Build history of the part. All positions in model axes, mm. Give positions to 0.01 mm unless a question says otherwise; leave off trailing zeros. Order: outer loops, then holes, each group sorted by start corner. A loop starts at its lowest first (then second) coordinate and runs counter-clockwise, first axis right, second up. Notation, with made-up numbers: (-19, -6.5) - (-2, -6.5) arc R29 cw to (-2, 21.5) - close; hole circle Ø4 at (12, -21). An arc over 180 degrees is marked (long way). Use a Markdown table: item, result.
from build123d import *

# Parameters (mm, degrees)
F0_R     = 34
F1_DEPTH = 0.5


with BuildPart() as f1:
    # F0 (on Top) → F1 (new body)
    with BuildSketch(Plane.XY):
        Circle(F0_R)
        with BuildLine():
            ThreePointArc((-27.595006, 7.125), (-22.1129, 10.357106), (-18.880794, 4.875))
            ThreePointArc((-18.880794, 4.875), (-19.5, 0), (-18.880794, -4.875))
            ThreePointArc((-18.880794, -4.875), (-22.1129, -10.357106), (-27.595006, -7.125))
            ThreePointArc((-27.595006, -7.125), (-28.5, 0), (-27.595006, 7.125))
        make_face(mode=Mode.SUBTRACT)
        with BuildLine():
            ThreePointArc((18.880794, -4.875), (19.5, 0), (18.880794, 4.875))
            ThreePointArc((18.880794, 4.875), (22.1129, 10.357106), (27.595006, 7.125))
            ThreePointArc((27.595006, 7.125), (28.5, 0), (27.595006, -7.125))
            ThreePointArc((27.595006, -7.125), (22.1129, -10.357106), (18.880794, -4.875))
        make_face(mode=Mode.SUBTRACT)
    extrude(amount=F1_DEPTH)


solid = f1.part
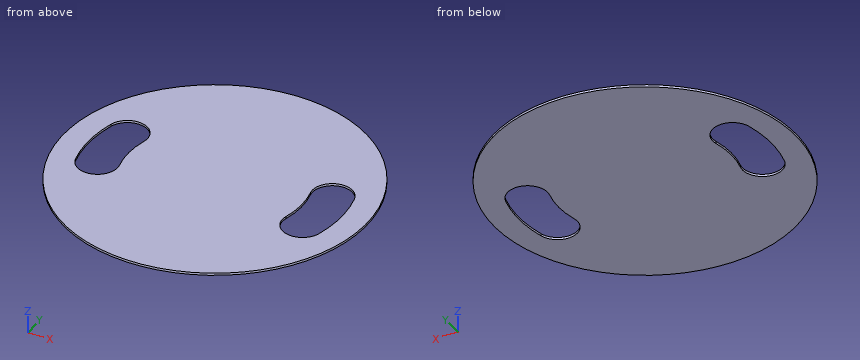
1) Slice it at D-D (x = 24). Write the cut outline in (y, z) (3 decimals), and give its area (3 significant figures).
Computed:
| item | result |
|---|---|
| outline | (-24.083, 0) - (-10.435, 0) - (-10.435, 0.5) - (-24.083, 0.5) - close; (10.435, 0) - (24.083, 0) - (24.083, 0.5) - (10.435, 0.5) - close |
| area | 13.6 mm² |
2) Pin check, flat tip, straight feed: P1, Ø6, axis at x = 19, y = 22.5, coming from the -Z side. Stop position of the tip, or through.
Computed:
| item | result |
|---|---|
| P1 | stops at z = 0 |
3) Slice it at A-A (z = 0.1). Write the cut outline in (x, y) (3 decimals), and give its area (3 significant figures).
Computed:
| item | result |
|---|---|
| outline | circle Ø68 at (0, 0); hole (-27.595, -7.125) arc R4.5 ccw to (-18.881, -4.875) arc R19.5 cw to (-18.881, 4.875) arc R4.5 ccw to (-27.595, 7.125) arc R28.5 ccw to start; hole (18.881, -4.875) arc R4.5 ccw to (27.595, -7.125) arc R28.5 ccw to (27.595, 7.125) arc R4.5 ccw to (18.881, 4.875) arc R19.5 cw to start |
| area | 3,290 mm² |
4) Slice it at C-C (x = -26). Write the cut outline in (y, z), and give its area (3 significant figures).
Computed:
| item | result |
|---|---|
| outline | (-21.91, 0) - (-9.55, 0) - (-9.55, 0.5) - (-21.91, 0.5) - close; (9.55, 0) - (21.91, 0) - (21.91, 0.5) - (9.55, 0.5) - close |
| area | 12.4 mm² |
5) Slice it at B-B (y = 0). Write the cut outline in (x, z).
Computed:
| item | result |
|---|---|
| outline | (-34, 0) - (-28.5, 0) - (-28.5, 0.5) - (-34, 0.5) - close; (-19.5, 0) - (19.5, 0) - (19.5, 0.5) - (-19.5, 0.5) - close; (28.5, 0) - (34, 0) - (34, 0.5) - (28.5, 0.5) - close |
6) Wall check: line 1 (X direction, y = 2, z = 0.4); line 2 (X direction, y = -1, z = 0.1); line 3 (Y direction, x = -25, z = 0.35). Give the ranges that are in metal, low to high. Write a range as from..to.
Computed:
| item | result |
|---|---|
| line 1 | x = -33.94..-28.43, -19.4..19.4, 28.43..33.94 |
| line 2 | x = -33.99..-28.48, -19.47..19.47, 28.48..33.99 |
| line 3 | y = -23.04..-10.14, 10.14..23.04 |
